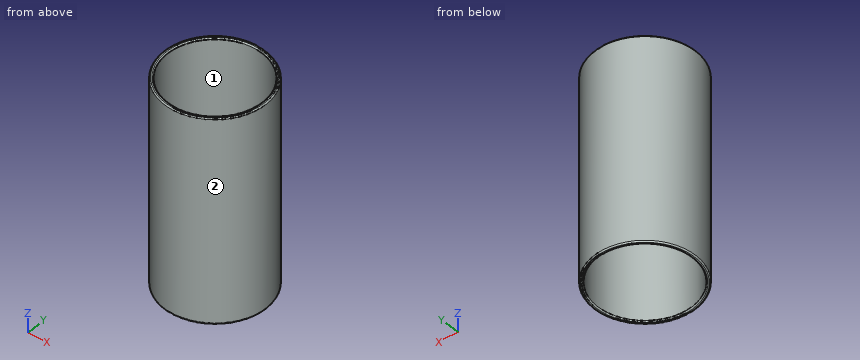
Autodesk Inventor part; units mm, degrees
ref_plane "YZ Plane" through (0, 0, 0) normal (1, 0, 0) x (0, 1, 0)
ref_plane "XZ Plane" through (0, 0, 0) normal (0, 1, 0) x (-1, 0, 0)
ref_plane "XY Plane" through (0, 0, 0) normal (0, 0, 1) x (1, 0, 0)
sketch "Sketch1" plane through (0, 0, 0) normal (0, 0, 1) x (1, 0, 0)
  circle A0 centre (0, 0) radius 44.7
  circle A1 centre (0, 0) radius 41.7
  dimension "d0" = 89.4
  dimension "d1" = 83.4
extrude "Extrusion1" add sketch "Sketch1" along normal blind 180
thread "Thread1"
fillet "Fillet1" radius 1 2 edges at (-44.7, 0, 180) (-41.7, 0, 180)
fillet "Fillet2" radius 1 2 edges at (-41.7, 0, 0) (-44.7, 0, 0)
properties part number "4111_Bias_Coil_Layer4_MPSv2_v2" material "Copper"
CAD build for the part. Positions are in the model's coordinates, mm. Face numbers are marked on the shaded views. Give positions to 0.01 mm unless a question says otherwise; leave off trailing zeros. Loops run counter-clockwise (first coordinate to the right, second up) from the corner with the lowest first, then second, coordinate; pieces in that order, holes last. Notation, with made-up numbers: M 65,66 L 123,66 A7 cw 123,74 Z; hole C 83,1 d8. An arc over 180 degrees is marked long. One line per question, with ' | ' between items. Start each with the question number.
1. Saw through at A-A on x = 0. Give the cut face in (y, z).
2. Saw through at C-C on z = 23.5. Give the cut face in (x, y), plus the area to 3 significant figures.
3. Probe L1, parallel to Y at x = 0, z = 87; L2, parallel to Y at x = 32.5, z = 15.5. List the from-to ranges inside material, lowest first. Write a range as from..to.
4. Flat gauge pins, fed straight in: pin 1 (1 mm diameter, centred on x = 19.5, z = 85.5, fed in from +Y); pin 2 (5 mm diameter, centred on x = -26.5, z = 96.5, fed in from -Y); pin 3 (12 mm diameter, centred on y = -35.5, z = 20, fed in from -X). Where does each tip first touch, or does it go through?
5. Two-plate mould, pull along Y, no slides. Class the marked faces 1 and 2: pulls with the +Y half, pulls with the -Y half, needs draft (parallel to the pull), parting line crosses it, or undercut.
Result sheet:
1) outline: M -44.7,1 A1 ccw -43.7,0 L -42.7,0 A1 ccw -41.7,1 L -41.7,179 A1 ccw -42.7,180 L -43.7,180 A1 ccw -44.7,179 Z; M 41.7,1 A1 ccw 42.7,0 L 43.7,0 A1 ccw 44.7,1 L 44.7,179 A1 ccw 43.7,180 L 42.7,180 A1 ccw 41.7,179 Z
2) outline: C 0,0 d89.4; hole C 0,0 d83.4 | area: 814 mm^2
3) L1: y = -44.7..-41.7, 41.7..44.7 | L2: y = -30.69..-26.13, 26.13..30.69
4) pin 1: stops at y = 40.46 | pin 2: stops at y = -37.71 | pin 3: stops at x = -33.58
5) face 1: undercut | face 2: parting line crosses it
